```python
from build123d import *

# Parameters (mm, degrees)
SKETCH1_R           = 1.5
BOSS_EXTRUDE1_DEPTH = 6.35
FILLET1_R           = 6.35
SKETCH2_R           = 1.5
CUT_EXTRUDE1_DEPTH  = 78.771299333


with BuildPart() as part:
    # Sketch1 → Boss-Extrude1 (new body)
    with BuildSketch(Plane.XY):
        with BuildLine():
            Line((0, 6.35), (-50.8, 6.35))
            Line((-50.8, 6.35), (-50.8, 44.45))
            Line((-50.8, 44.45), (-63.5, 44.45))
            Line((-63.5, 44.45), (-63.5, -6.35))
            Line((-63.5, -6.35), (0, -6.35))
            ThreePointArc((0, -6.35), (6.35, 0), (0, 6.35))
        make_face()
        Circle(SKETCH1_R, mode=Mode.SUBTRACT)
    extrude(amount=BOSS_EXTRUDE1_DEPTH)

    # Fillet1
    fillet1_edges = [part.edges().sort_by_distance(p)[0] for p in [
        (-63.5, -6.35, 3.175),
        (-50.8, 6.35, 3.175),
        (-63.5, 44.45, 3.175),
        (-50.8, 44.45, 3.175),
    ]]
    fillet(fillet1_edges, radius=FILLET1_R - 0.0001)  # a hair under: the kernel refuses the full size

    # Sketch2 → Cut-Extrude1 (cut, through all)
    with BuildSketch(Plane(origin=(0, 0, 0), x_dir=(-1, 0, 0), z_dir=(0, 0, -1))):
        with Locations((6.35, 0)):
            Circle(SKETCH2_R)
        with Locations((12.7, 0)):
            Circle(SKETCH2_R)
        with Locations((25.4, 0)):
            Circle(SKETCH2_R)
        with Locations((19.05, 0)):
            Circle(SKETCH2_R)
    extrude(amount=-CUT_EXTRUDE1_DEPTH, mode=Mode.SUBTRACT)


solid = part.part
```
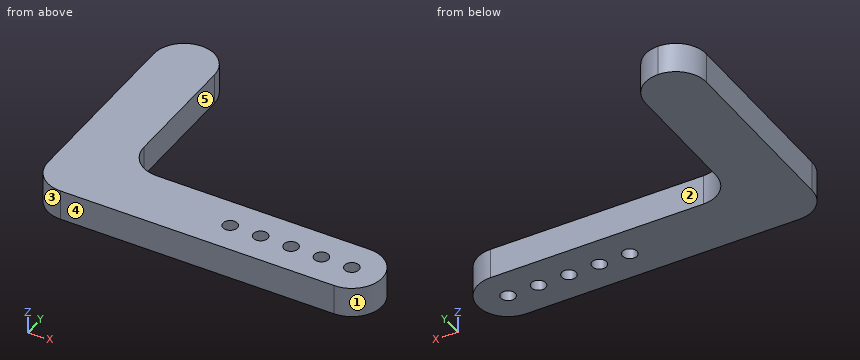
Model file for the job. Use its own axes, mm. Face numbers are marked on the shaded views. A direction names the side the tool comes from. Give positions to 0.01 mm unless a question says otherwise; leave off trailing zeros. Order: outer loops, then holes, each group sorted by start corner. A loop starts at its lowest first (then second) coordinate and runs counter-clockwise, first axis right, second up.
1) Saw through at A-A, the plane x = -19.05. Write the cut outline in (y, z), then the cut area to 3 significant figures.
2) Pin check, flat tips, straight feed: pin 1 (1.5 mm diameter, centred on y = 37.5, z = 3.5, fed in from +X); pin 2 (1.9 mm diameter, centred on x = -22, z = 3.5, fed in from +Y); pin 3 (2.5 mm diameter, centred on x = -12.7, y = 0, fed in from -Z). Stop position of each tip, or through.
3) 3-axis set-ups, long thin cutter, end or side, ignore diameter. For the marked faces 1 and 2: which of +Z, -Z, +X, -X, +Y, -Y reach the whole face in a straight line?
4) Saw through at C-C, the plane y = 22.5. Write the cut outline in (x, z), then the cut area to 3 significant figures.
5) Mould opens along X. For the marked faces 3, 4 and 5 say: +X half, -X half, draft (parallel to the pull), parting line (faces both ways), or undercut.
6) Saw through at B-B, the plane z = 4.75. Count the separate pieces of the cut face and the enclosed holes in it, then the cut area to 3 significant figures.
7) Wall check: probe 1 along Y at (x, z) = (-12.5, 2.25); probe 2 along X at (y, z) = (25, 4); probe 3 along Y at (x, z) = (-30, 0.5). Give the ranges that are in metal, low to high.
8) Saw through at D-D, the plane x = -35. Write the cut outline in (y, z).
Computed:
1. outline: (-6.35, 0) - (-1.5, 0) - (-1.5, 6.35) - (-6.35, 6.35) - close; (1.5, 0) - (6.35, 0) - (6.35, 6.35) - (1.5, 6.35) - close
1. area: 61.6 mm2
2. pin 1: stops at x = -50.8
2. pin 2: stops at y = 6.35
2. pin 3: passes through
3. face 1: +Z, -Z, +X
3. face 2: +Z, -Z, +X, +Y
4. outline: (-63.5, 0) - (-50.8, 0) - (-50.8, 6.35) - (-63.5, 6.35) - close
4. area: 80.6 mm2
5. face 3: -X half
5. face 4: draft
5. face 5: +X half
6. separate pieces: 1
6. enclosed holes: 5
6. area: 1,300 mm2
7. probe 1: y = -6.35 to -1.49, 1.49 to 6.35
7. probe 2: x = -63.5 to -50.8
7. probe 3: y = -6.35 to 6.35
8. outline: (-6.35, 0) - (6.35, 0) - (6.35, 6.35) - (-6.35, 6.35) - close
